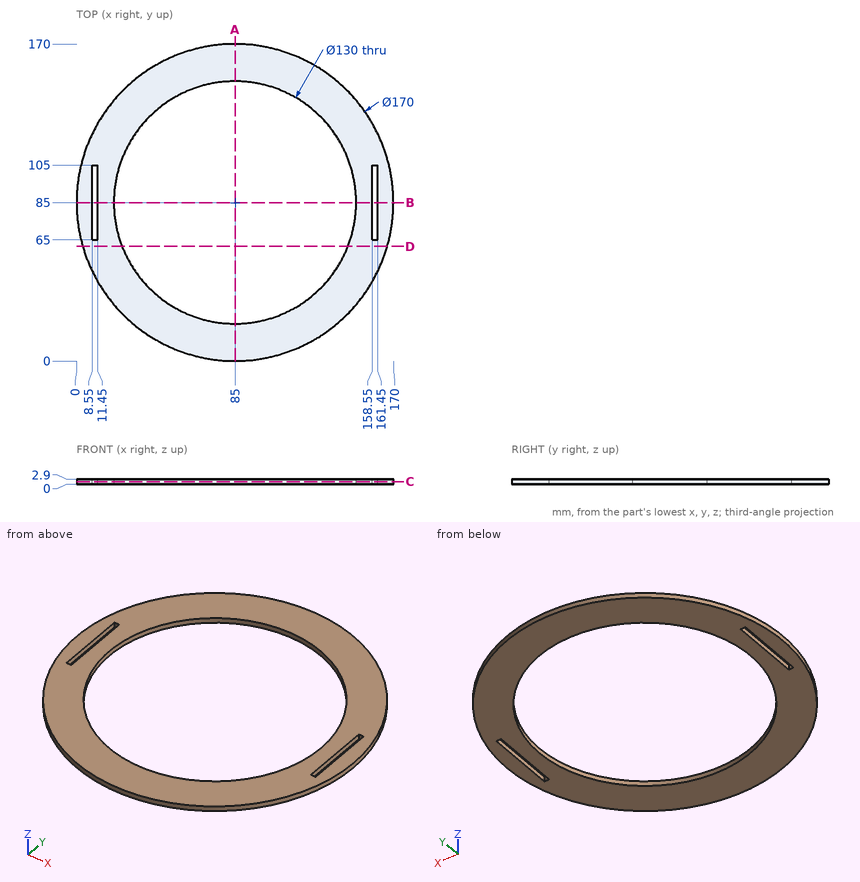
Geometry check sheet. Reference: drawing and pictorial views, mm from the part's lowest x, y, z. Give positions to 0.01 mm unless a question says otherwise; leave off trailing zeros. Write each loop counter-clockwise with the first axis right and the second up, starting at its lowest first coordinate (ties: lowest second). Pieces come first, ordered by that corner, then holes. Notation, with made-up numbers: (0, -20.75) -> (21, -20.75) arc R12 cw to (21, -10.75) -> close; hole circle Ø10 at (-20, 59.25). An arc over 180 degrees is marked (long way). One line per question, with ' | ' between items.
Item 1: Sectioned sample at A-A, the plane x = 85. Record the boundary of the cut face in (y, z), plus the area to 3 significant figures.
Determined:
outline: (0, 0) -> (20, 0) -> (20, 2.9) -> (0, 2.9) -> close; (150, 0) -> (170, 0) -> (170, 2.9) -> (150, 2.9) -> close | area: 116 mm^2
Item 2: Scan lines: line 1 along X through (y, z) = (87, 2); line 2 along Y through (x, z) = (85, 1.55); line 3 along X through (y, z) = (75.5, 0.2). Record each from-to range of solid material in increasing order.
Determined:
line 1: 0.02 to 8.55, 11.45 to 20.03, 149.97 to 158.55, 161.45 to 169.98 | line 2: 0 to 20, 150 to 170 | line 3: 0.53 to 8.55, 11.45 to 20.7, 149.3 to 158.55, 161.45 to 169.47
Item 3: Sectioned sample at C-C, the plane z = 1.5. Record the boundary of the cut face in (x, y).
Determined:
outline: circle Ø170 at (85, 85); hole (8.55, 65) -> (11.45, 65) -> (11.45, 105) -> (8.55, 105) -> close; hole circle Ø130 at (85, 85); hole (158.55, 65) -> (161.45, 65) -> (161.45, 105) -> (158.55, 105) -> close
Item 4: Sectioned sample at B-B, the plane y = 85. Record the boundary of the cut face in (x, z).
Determined:
outline: (0, 0) -> (8.55, 0) -> (8.55, 2.9) -> (0, 2.9) -> close; (11.45, 0) -> (20, 0) -> (20, 2.9) -> (11.45, 2.9) -> close; (150, 0) -> (158.55, 0) -> (158.55, 2.9) -> (150, 2.9) -> close; (161.45, 0) -> (170, 0) -> (170, 2.9) -> (161.45, 2.9) -> close
Item 5: Depth check by flat-ended pin: pin 1 (1.5 mm diameter, centred on y = 106, z = 1, fed in from +X); pin 2 (1.4 mm diameter, centred on y = 82.5, z = 1.5, fed in from +X); pin 3 (0.9 mm diameter, centred on y = 77, z = 1.5, fed in from -X). Enter the tip coordinate at first touch or a pass-through.
Determined:
pin 1: x = 167.55 | pin 2: x = 169.98 | pin 3: x = 0.34
Item 6: Sectioned sample at D-D, the plane y = 61.5. Record the boundary of the cut face in (x, z), plus the area to 3 significant figures.
Determined:
outline: (3.31, 0) -> (24.4, 0) -> (24.4, 2.9) -> (3.31, 2.9) -> close; (145.6, 0) -> (166.69, 0) -> (166.69, 2.9) -> (145.6, 2.9) -> close | area: 122 mm^2
